from build123d import *

# Parameters (mm, degrees)
F1_DEPTH = 18
F3_D     = 6.5
F3_DEPTH = 25
F3_TIP   = 1.9527970118


# Not quite as in the source:
# - a feature names something its author has since deleted; it is built from what else it names


with BuildPart() as f1:
    # F0 (on Front) → F1 (new body)
    with BuildSketch(Plane.XZ):
        with BuildLine():
            Line((0, 0), (0, -100))
            Line((0, -100), (-90, -730))
            Line((-90, -730), (-30, -730))
            Line((-30, -730), (119, -100))
            Line((119, -100), (119, -55))
            Line((119, -55), (103, -55))
            Line((103, -55), (103, -25))
            Line((103, -25), (103, 0))
            Line((103, 0), (78.25, 0))
            Line((78.25, 0), (78.25, -47))
            ThreePointArc((78.25, -47), (80.3713203436, -52.1213203436), (75.25, -50))
            Line((75.25, -50), (62.75, -50))
            ThreePointArc((62.75, -50), (57.6286796564, -52.1213203436), (59.75, -47))
            Line((59.75, -47), (59.75, 0))
            Line((59.75, 0), (0, 0))
        make_face()
    extrude(amount=F1_DEPTH)

    # F3
    with Locations(Plane.YZ.offset(103)):
        with Locations((-9, -25)):
            Hole(F3_D / 2, depth=F3_DEPTH)
            with Locations((0, 0, -(F3_DEPTH + F3_TIP / 2))):  # 118° drill point
                Cone(0, F3_D / 2, F3_TIP, mode=Mode.SUBTRACT)


solid = f1.part
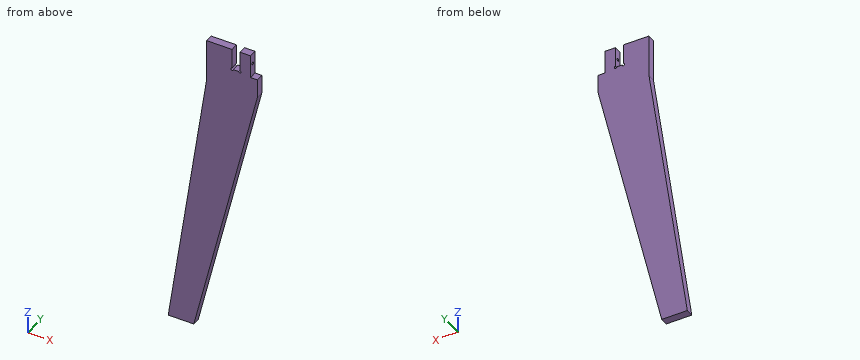
Part model, mm, in its own coordinate system. Give positions to 0.01 mm unless a question says otherwise; leave off trailing zeros. Loops run counter-clockwise (first coordinate to the right, second up) from the corner with the lowest first, then second, coordinate; pieces in that order, holes last. Notation, with made-up numbers: M 33.25,3.5 L 44.25,3.5 A25 cw 44.25,25.5 Z; hole C 84.5,25.25 d10. An arc over 180 degrees is marked long. Put each result on its own line as item: value. Start each with the question number.
1) Flat gauge pins, fed straight in: pin 1 (5.5 mm diameter, centred on y = -12.5, z = -15.5, fed in from +X); pin 2 (4 mm diameter, centred on y = -9.5, z = -360.5, fed in from +X); pin 3 (5.5 mm diameter, centred on x = 59.75, z = -50, fed in from +Y); pin 4 (8 mm diameter, centred on y = -12.5, z = -420.5, fed in from +X). Where does each tip first touch, or does it go through?
2) Saw through at C-C (x = 36). List the corners of the cut face in (y, z), then the cut area to 3 significant figures.
3) Probe probe 1 along X at (y, z) = (-16.75, -41.5); probe 2 along X at (y, z) = (-7.75, -332.5); probe 3 along X at (y, z) = (-3.75, -115). List the from-to ranges inside material, lowest first.
4) Saw through at A-A (y = -9). List the corners of the cut face in (x, z), then the cut area to 3 significant figures.
5) Saw through at B-B (z = -144). List the corners of the cut face in (x, y).
Numbers:
1. pin 1: x = 103
1. pin 2: x = 57.86
1. pin 3: through
1. pin 4: x = 44.15
2. outline: M -18,-450.94 L 0,-450.94 L 0,0 L -18,0 Z
2. area: 8,120 mm^2
3. probe 1: 0 to 59.75, 78.25 to 103
3. probe 2: -33.21 to 64.01
3. probe 3: -2.14 to 115.45
4. outline: M -90,-730 L -30,-730 L 119,-100 L 119,-55 L 103,-55 L 103,-28.25 L 78.25,-28.25 L 78.25,-47 A3 cw long 75.25,-50 L 62.75,-50 A3 cw long 59.75,-47 L 59.75,0 L 0,0 L 0,-100 Z; M 78.25,-21.75 L 103,-21.75 L 103,0 L 78.25,0 Z
4. area: 66,300 mm^2
5. outline: M -6.29,-18 L 108.59,-18 L 108.59,0 L -6.29,0 Z
